Design review of the part built by this model. Coordinates are the model's own, in mm. A direction names the side the tool comes from. Round coordinates to 2 decimals unless told otherwise and drop trailing zeros. Write each loop counter-clockwise with the first axis right and the second up, starting at its lowest first coordinate (ties: lowest second). Pieces come first, ordered by that corner, then holes.
from build123d import *

# Parameters (mm, degrees)
EXTRUDE_1_DEPTH     = 32
SKETCH_2_R          = 2.1
CUT_EXTRUDE_1_DEPTH = 5
SKETCH_3_W          = 6
SKETCH_3_H          = 6
SKETCH_3_H_2        = 32
SKETCH_3_H_3        = 43
CUT_EXTRUDE_2_DEPTH = 6
SKETCH_4_R          = 1
CUT_EXTRUDE_3_DEPTH = 38
CUT_EXTRUDE_4_DEPTH = 289.729583292


with BuildPart() as part:
    # 草图1 → 凸台-拉伸1 (new body)
    with BuildSketch(Plane.XY):
        with BuildLine():
            Line((194.787878788, 116.363636364), (200.787878788, 116.363636364))
            Line((200.787878788, 116.363636364), (200.787878788, -78.636363636))
            ThreePointArc((200.787878788, -78.636363636), (197.8589466, -85.707431448), (190.787878788, -88.636363636))
            Line((190.787878788, -88.636363636), (-79.212121212, -88.636363636))
            ThreePointArc((-79.212121212, -88.636363636), (-86.283189024, -85.707431448), (-89.212121212, -78.636363636))
            Line((-89.212121212, -78.636363636), (-89.212121212, 116.363636364))
            Line((-89.212121212, 116.363636364), (-81.212121212, 116.363636364))
            Line((-81.212121212, 116.363636364), (-81.212121212, -70.636363636))
            ThreePointArc((-81.212121212, -70.636363636), (-78.283189024, -77.707431448), (-71.212121212, -80.636363636))
            Line((-71.212121212, -80.636363636), (184.787878788, -80.636363636))
            ThreePointArc((184.787878788, -80.636363636), (191.8589466, -77.707431448), (194.787878788, -70.636363636))
            Line((194.787878788, -70.636363636), (194.787878788, 116.363636364))
        make_face()
    extrude(amount=EXTRUDE_1_DEPTH)

    # 草图2 → 切除-拉伸1 (cut)
    with BuildSketch(Plane(origin=(0, 0, 0), x_dir=(-1, 0, 0), z_dir=(0, 0, -1))):
        with Locations((-182.787878788, -84.636363636)):
            Circle(SKETCH_2_R)
        with Locations((-55.787878788, -84.636363636)):
            Circle(SKETCH_2_R)
        with Locations((71.212121212, -84.636363636)):
            Circle(SKETCH_2_R)
    extrude(amount=-CUT_EXTRUDE_1_DEPTH, mode=Mode.SUBTRACT)

    # 草图3 → 切除-拉伸2 (cut)
    with BuildSketch(Plane.ZY.offset(89.212121212)):
        with Locations((29, -5.636363636)):
            Rectangle(SKETCH_3_W, SKETCH_3_H)
        with Locations((29, 16.363636364)):
            Rectangle(SKETCH_3_W, SKETCH_3_H_2)
        with Locations((29, 56.863636364)):
            Rectangle(SKETCH_3_W, SKETCH_3_H_3)
    extrude(amount=-CUT_EXTRUDE_2_DEPTH, mode=Mode.SUBTRACT)

    # 草图4 → 切除-拉伸3 (cut)
    with BuildSketch(Plane(origin=(0, 35.363636364, 0), x_dir=(1, 0, 0), z_dir=(0, 1, 0))):
        with Locations(Location((-87.212121212, -29, 0), (0, 0, 270))):
            Circle(SKETCH_4_R)
    extrude(amount=-CUT_EXTRUDE_3_DEPTH, mode=Mode.SUBTRACT)

    # 草图6 → 切除-拉伸4 (cut, through all)
    with BuildSketch(Plane.XZ.offset(88.636363636)):
        with BuildLine():
            Line((-89.212121212, 32), (-85.912121212, 32))
            ThreePointArc((-85.912121212, 32), (-88.24557359, 31.033452378), (-89.212121212, 28.7))
            Line((-89.212121212, 28.7), (-89.212121212, 32))
        make_face()
    extrude(amount=-CUT_EXTRUDE_4_DEPTH, mode=Mode.SUBTRACT)


solid = part.part
1) Add section B-B on z = 18. State the section outline as (x, y) points, and give its area (3 significant figures).
2) Add section A-A on y = 43. State the section outline as (x, z) points.
3) For faces 1 (the face through (-86, 16, 26)), 2 (the face through (-86.21, -85.78, 15.78)), 3 (the face through (191.781, -77.785, 15.776)), list the 3-axis set-ups (+Z, -Z, +X, -X, +Y, -Y) from which the entire face can be reached by the end or side of a thin tool; tool diameter is ignored.
4) Add section D-D on x = 22. State the section outline as (y, z) points, and give its area (3 significant figures).
5) Add section C-C on y = -29.5. State the section outline as (x, z) points, and give its area (3 significant figures).
6) For line 1 along X through (y, z) = (33.45, 29); line 2 along X through (y, z) = (60, 24); line 3 along Y through (x, z) = (27, 9), list the stretches that pass through material, from the lowest coordinate up.
7) For P1, Ø2, axis at x = 56, y = -85.5, coming from the -Z side; P2, Ø3, axis at y = -6, z = 28.5, coming from the -X side; P3, Ø6, axis at x = 72.5, z = 11.5, coming from the +Y side, all flat-tipped, find the tip position at first contact; note any pin that passes through.
8) The part is to be moulded in two halves that separate along Y. For faces 4 (the face through (198, 116.364, 16)), 5 (the face through (-86, 57, 26)), 6 (the face through (-81.212, 24, 16)), say which applies: pulls with the +Y half, pulls with the -Y half, needs draft (parallel to the pull), parting line crosses it, or undercut.
Computed:
1. outline: (-89.21, -78.64) arc R10 ccw to (-79.21, -88.64) - (190.79, -88.64) arc R10 ccw to (200.79, -78.64) - (200.79, 116.36) - (194.79, 116.36) - (194.79, -70.64) arc R10 cw to (184.79, -80.64) - (-71.21, -80.64) arc R10 cw to (-81.21, -70.64) - (-81.21, 116.36) - (-89.21, 116.36) - close
1. area: 5,080 mm2
2. outline: (-89.21, 0) - (-81.21, 0) - (-81.21, 32) - (-83.21, 32) - (-83.21, 26) - (-89.21, 26) - close; (194.79, 0) - (200.79, 0) - (200.79, 32) - (194.79, 32) - close
3. face 1: +Z, -X
3. face 2: +Z, -Z, -X, -Y
3. face 3: +Z, -Z, +Y
4. outline: (-88.64, 0) - (-80.64, 0) - (-80.64, 32) - (-88.64, 32) - close
4. area: 256 mm2
5. outline: (-89.21, 0) - (-81.21, 0) - (-81.21, 32) - (-85.91, 32) arc R3.3 ccw to (-89.21, 28.7) - close; (194.79, 0) - (200.79, 0) - (200.79, 32) - (194.79, 32) - close
5. area: 446 mm2
6. line 1: x = -89.2 to -88.21, -86.21 to -81.21, 194.79 to 200.79
6. line 2: x = -89.21 to -81.21, 194.79 to 200.79
6. line 3: y = -88.64 to -80.64
7. P1: stops at z = 5
7. P2: stops at x = -83.21
7. P3: stops at y = -80.64
8. face 4: pulls with the +Y half
8. face 5: undercut
8. face 6: needs draft
